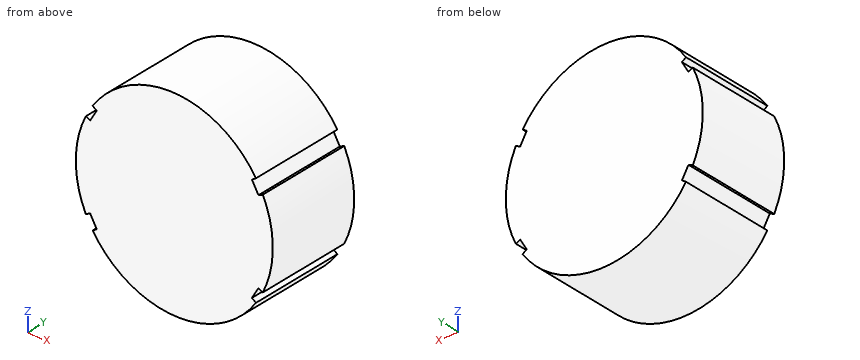
```python
from build123d import *

# Parameters (mm, degrees)
BOSS_EXTRUDE1_DEPTH = 24


with BuildPart() as part:
    # Sketch1 → Boss-Extrude1 (new body)
    with BuildSketch(Plane(origin=(0, 0, 0), x_dir=(1, 0, 0), z_dir=(0, 1, 0))):
        with BuildLine():
            Line((21.34980207, 10.421058084), (19.69980207, 13.278941916))
            Line((19.69980207, 13.278941916), (20.730203224, 13.973499))
            ThreePointArc((20.730203224, 13.973499), (0, 25), (-20.730203224, 13.973499))
            Line((-20.730203224, 13.973499), (-19.69980207, 13.278941916))
            Line((-19.69980207, 13.278941916), (-21.34980207, 10.421058084))
            Line((-21.34980207, 10.421058084), (-22.466506726, 10.966133117))
            ThreePointArc((-22.466506726, 10.966133117), (-25, 0), (-22.466506726, -10.966133117))
            Line((-22.466506726, -10.966133117), (-21.34980207, -10.421058084))
            Line((-21.34980207, -10.421058084), (-19.69980207, -13.278941916))
            Line((-19.69980207, -13.278941916), (-20.730203224, -13.973499))
            ThreePointArc((-20.730203224, -13.973499), (0, -25), (20.730203224, -13.973499))
            Line((20.730203224, -13.973499), (19.69980207, -13.278941916))
            Line((19.69980207, -13.278941916), (21.34980207, -10.421058084))
            Line((21.34980207, -10.421058084), (22.466506726, -10.966133117))
            ThreePointArc((22.466506726, -10.966133117), (25, 0), (22.466506726, 10.966133117))
            Line((22.466506726, 10.966133117), (21.34980207, 10.421058084))
        make_face()
    extrude(amount=BOSS_EXTRUDE1_DEPTH)


solid = part.part
```
Source: CAD feature listing. Evaluate the final solid. Frame: model axes, mm. Coordinates: 2 decimals unless noted, no trailing zeros. Loops run counter-clockwise (first coordinate to the right, second up) from the corner with the lowest first, then second, coordinate; pieces in that order, holes last. Notation, with made-up numbers: M 78,44.5 L 134,44.5 A18 cw 134,52.5 Z; hole C 62,68.5 d5. An arc over 180 degrees is marked long. Put each result on its own line as item: value. Start each with the question number.
1) Cut plane B-B on x = 15. Return the cut outline in (y, z), then the cut area to 3 significant figures.
2) Contact query for flat-ended pins moving along their axis: pin 1 Ø8 at (x, y) = (-9.5, 17) entering from -Z; pin 2 Ø1.5 at (x, y) = (-16, 3.5) entering from -Z; pin 3 Ø3 at (x, y) = (-5.5, 11.5) entering from +Z. Output: stop coordinate, or through.
3) Ray query, L1, parallel to Z at x = 20.5, y = 10.5; L2, parallel to Z at x = -10, y = 6; L3, parallel to X at y = 20.5, z = -12.5. Return the intervals inside material, ascending. Write a range as from..to.
4) Cut plane C-C on z = -20. Return the cut outline in (x, y), then the cut area to 3 significant figures.
5) Cut plane A-A on y = 2.75. Return the cut outline in (x, z), then the cut area to 3 significant figures.
The answers:
1. outline: M 0,-20 L 24,-20 L 24,20 L 0,20 Z
1. area: 960 mm²
2. pin 1: stops at z = -24.39
2. pin 2: stops at z = -19.81
2. pin 3: stops at z = 24.68
3. L1: z = -14.31..-13.82, -11.89..11.89, 13.82..14.31
3. L2: z = -22.91..22.91
3. L3: x = -20.15..20.15
4. outline: M -15,0 L 15,0 L 15,24 L -15,24 Z
4. area: 720 mm²
5. outline: M -22.47,-10.97 L -21.35,-10.42 L -19.7,-13.28 L -20.73,-13.97 A25 ccw 20.73,-13.97 L 19.7,-13.28 L 21.35,-10.42 L 22.47,-10.97 A25 ccw 22.47,10.97 L 21.35,10.42 L 19.7,13.28 L 20.73,13.97 A25 ccw -20.73,13.97 L -19.7,13.28 L -21.35,10.42 L -22.47,10.97 A25 ccw Z
5. area: 1,950 mm²
